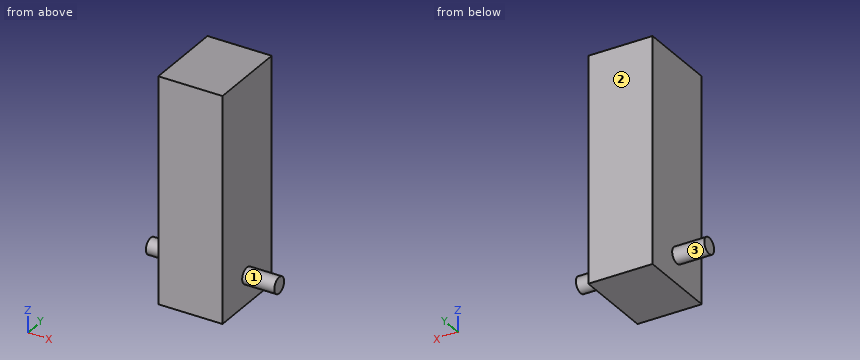
```python
from build123d import *

# Parameters (mm, degrees)
SKETCH_1_W             = 20
SKETCH_1_H             = 70
EXTRUDE_326_DEPTH      = 25
SKETCH_2_R             = 2.5
EXTRUDE_591_DEPTH      = 10
EXTRUDE_591_DEPTH_BACK = 30


with BuildPart() as part:
    # Эскиз1 → Extrude 326 (new body)
    with BuildSketch(Plane(origin=(0, 0, 0), x_dir=(1, 0, 0), z_dir=(0, 1, 0))):
        with Locations((-10, 35)):
            Rectangle(SKETCH_1_W, SKETCH_1_H)
    extrude(amount=EXTRUDE_326_DEPTH)

    # Эскиз2 → Extrude 591 (add, two sides)
    with BuildSketch(Plane(origin=(0, 0, 0), x_dir=(0, 0, -1), z_dir=(1, 0, 0))) as extrude_591_sk:
        with Locations((61.25, 12.5)):
            Circle(SKETCH_2_R)
    extrude(amount=EXTRUDE_591_DEPTH)
    extrude(extrude_591_sk.sketch, amount=-EXTRUDE_591_DEPTH_BACK)


solid = part.part
```
Geometry: final body of the model. Coordinates: model frame, mm. Face numbers are marked on the shaded views. A direction names the side the tool comes from. Coordinates: 2 decimals unless noted, no trailing zeros. Order: outer loops, then holes, each group sorted by start corner. A loop starts at its lowest first (then second) coordinate and runs counter-clockwise, first axis right, second up. Notation, with made-up numbers: (48.25, 33) -> (65.25, 33) arc R21 cw to (65.25, 54) -> close; hole circle Ø4 at (-13.5, -36). An arc over 180 degrees is marked (long way). Write each question's results on one line, items separated by ' | '. Start each with the question number.
1) Set-up query: the marked faces 1, 2 and 3. Return all of +Z, -Z, +X, -X, +Y, -Y with unobstructed straight access to the full face (end or side cutting, diameter ignored); none if empty.
2) First-contact query: pin 1 (1 mm diameter, centred on y = 8, z = -16.5, fed in from -X); pin 2 (5 mm diameter, centred on x = -25, y = 15, fed in from +Z); pin 3 (12.5 mm diameter, centred on y = 10.5, z = -34.5, fed in from +X). Flat tips, straight axial feed; report the tip coordinate or a pass-through.
3) Cut plane C-C, the plane x = -26. Output: boundary loops of the cut face in (y, z), and give its area (3 significant figures).
4) Cut plane A-A, the plane z = -61.25. Output: boundary loops of the cut face in (x, y), and give its area (3 significant figures).
5) Cut plane B-B, the plane y = 12.5. Output: boundary loops of the cut face in (x, z), and give its area (3 significant figures).
6) Cut plane D-D, the plane y = 16.75. Output: boundary loops of the cut face in (x, z), and give its area (3 significant figures).
7) Material intervals for line 1 along X through (y, z) = (20.5, -9), sorted ascending.
Checks:
1) face 1: +X | face 2: +Z, -Z, +X, -X, +Y | face 3: -X
2) pin 1: x = -20 | pin 2: z = -58.75 | pin 3: x = 0
3) outline: circle Ø5 at (12.5, -61.25) | area: 19.6 mm^2
4) outline: (-30, 10) -> (-20, 10) -> (-20, 0) -> (0, 0) -> (0, 10) -> (10, 10) -> (10, 15) -> (0, 15) -> (0, 25) -> (-20, 25) -> (-20, 15) -> (-30, 15) -> close | area: 600 mm^2
5) outline: (-30, -63.75) -> (-20, -63.75) -> (-20, -70) -> (0, -70) -> (0, -63.75) -> (10, -63.75) -> (10, -58.75) -> (0, -58.75) -> (0, 0) -> (-20, 0) -> (-20, -58.75) -> (-30, -58.75) -> close | area: 1,500 mm^2
6) outline: (-20, -70) -> (0, -70) -> (0, 0) -> (-20, 0) -> close | area: 1,400 mm^2
7) line 1: -20 to 0
